Read the model definition and answer for the solid it produces. Units are mm, in the model's axes. Face numbers are marked on the shaded views. A direction names the side the tool comes from. Coordinates: 2 decimals unless noted, no trailing zeros. Loops run counter-clockwise (first coordinate to the right, second up) from the corner with the lowest first, then second, coordinate; pieces in that order, holes last. Notation, with made-up numbers: (49.25, 30) -> (93.25, 30) arc R26 cw to (93.25, 45) -> close; hole circle Ø3 at (58.5, 59.5). An arc over 180 degrees is marked (long way). Answer as a JSON object with one key per item and string values. Group by question number.
Q1. For the marked faces 1, 2 and 3, determine the directions among +Z, -Z, +X, -X, +Y, -Y from which every point of the face is accessible in a straight line to the end or side of a thin tool.
Q2. The part is cut by section A-A on y = 1. Write down the section's boundary in (x, z).
Q3. The part is cut by section D-D on z = 25.5. Write down the section's boundary in (x, y), and give its area (3 significant figures).
Q4. The part is cut by section C-C on x = 0. Write down the section's boundary in (y, z), and give its area (3 significant figures).
Q5. Straight lines are drawn through the part: line 1 along X through (y, z) = (2.45, 2.5); line 2 along Z through (x, y) = (1.75, 1.25); line 3 along X through (y, z) = (0.75, 23). For each, find the intervals that lie inside material, in ascending order. Write a range as [from, to].
Q6. The part is cut by section B-B on z = 9. Write down the section's boundary in (x, y), and give its area (3 significant figures).
Q7. Each of these flat-tipped pins is pushed along its axis until it touches: P1, Ø1.5, axis at x = 8, y = 4, coming from the +Z side; P2, Ø1.2, axis at x = 0, z = 2.5, coming from the +Y side; P3, Ø2.5, axis at y = 4.5, z = 19.5, coming from the -X side; P4, Ø1.5, axis at y = 4, z = 17, coming from the +X side. Where does it stop, or does it pass through?
Q8. Determine the mould class of the marked faces 4, 5 and 6 for opening direction X: released by +X, released by -X, zero draft, split by the parting line, or undercut.
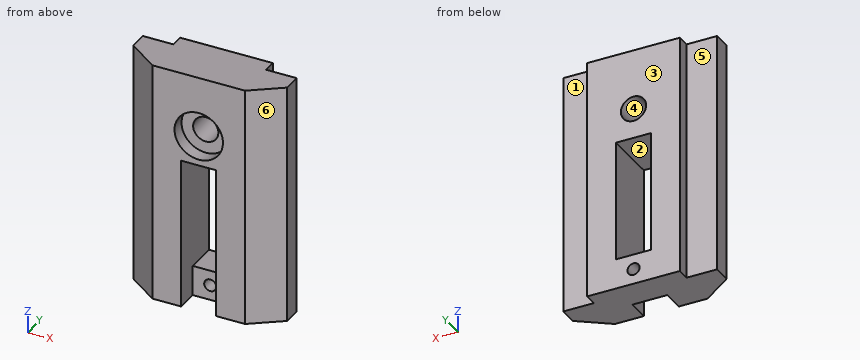
from build123d import *

# Parameters (mm, degrees)
BOSS_EXTRUDE1_DEPTH = 40
SKETCH2_R           = 2.0828
SKETCH2_R_2         = 1
CUT_EXTRUDE1_DEPTH  = 43.867462538
SKETCH3_W           = 5.776667402
SKETCH3_H           = 20
CUT_EXTRUDE2_DEPTH  = 43.867462538
SKETCH4_W           = 5.776667402
SKETCH4_H           = 5
CUT_EXTRUDE3_DEPTH  = 3.62
SKETCH5_R           = 4.0005
CUT_EXTRUDE4_DEPTH  = 2.2098


with BuildPart() as part:
    # Sketch1 → Boss-Extrude1 (new body)
    with BuildSketch(Plane.XY):
        Polygon((-7.65, 5.116666667), (7.65, 5.116666667), (7.65, 3), (12.7, 3), (12.7, 0), (7.65, -3.62), (-7.65, -3.62), (-12.7, 0), (-12.7, 3), (-7.65, 3), align=None)
    extrude(amount=BOSS_EXTRUDE1_DEPTH)

    # Sketch2 → Cut-Extrude1 (cut, through all)
    with BuildSketch(Plane.XZ.offset(3.62)):
        with Locations(Location((0, 30, 0), (0, 0, 270))):
            Circle(SKETCH2_R)
        with Locations(Location((0, 2.5, 0), (0, 0, 270))):
            Circle(SKETCH2_R_2)
    extrude(amount=-CUT_EXTRUDE1_DEPTH, mode=Mode.SUBTRACT)

    # Sketch3 → Cut-Extrude2 (cut, through all)
    with BuildSketch(Plane.XZ.offset(3.62)):
        with Locations((0, 15)):
            Rectangle(SKETCH3_W, SKETCH3_H)
    extrude(amount=-CUT_EXTRUDE2_DEPTH, mode=Mode.SUBTRACT)

    # Sketch4 → Cut-Extrude3 (cut)
    with BuildSketch(Plane.XZ.offset(3.62)):
        with Locations((0, 2.5)):
            Rectangle(SKETCH4_W, SKETCH4_H)
    extrude(amount=-CUT_EXTRUDE3_DEPTH, mode=Mode.SUBTRACT)

    # Sketch5 → Cut-Extrude4 (cut)
    with BuildSketch(Plane.XZ.offset(3.62)):
        with Locations(Location((0, 30, 0), (0, 0, 270))):
            Circle(SKETCH5_R)
    extrude(amount=-CUT_EXTRUDE4_DEPTH, mode=Mode.SUBTRACT)


solid = part.part
Final values:
{
 "1": {"face 1": "+Z, -Z, +X, +Y", "face 2": "+Y, -Y", "face 3": "+Z, -Z, +X, -X, +Y"},
 "2": {"outline": "(-12.7, 0) -> (12.7, 0) -> (12.7, 40) -> (-12.7, 40) -> close; hole (-2.89, 5) -> (2.89, 5) -> (2.89, 25) -> (-2.89, 25) -> close; hole circle Ø4.17 at (0, 30); hole circle Ø2 at (0, 2.5)"},
 "3": {"outline": "(-12.7, 0) -> (-7.65, -3.62) -> (7.65, -3.62) -> (12.7, 0) -> (12.7, 3) -> (7.65, 3) -> (7.65, 5.12) -> (-7.65, 5.12) -> (-7.65, 3) -> (-12.7, 3) -> close", "area": "182 mm2"},
 "4": {"outline": "(-3.62, 25) -> (5.12, 25) -> (5.12, 27.92) -> (-1.41, 27.92) -> (-1.41, 26) -> (-3.62, 26) -> close; (-3.62, 34) -> (-1.41, 34) -> (-1.41, 32.08) -> (5.12, 32.08) -> (5.12, 40) -> (-3.62, 40) -> close; (0, 0) -> (5.12, 0) -> (5.12, 1.5) -> (0, 1.5) -> close; (0, 3.5) -> (5.12, 3.5) -> (5.12, 5) -> (0, 5) -> close", "area": "102 mm2"},
 "5": {"line 1": "x = [-12.7, -1], [1, 12.7]", "line 2": "z = [0, 5], [25, 28.87], [31.13, 40]", "line 3": "x = [-12.7, -2.89], [2.89, 12.7]"},
 "6": {"outline": "(-12.7, 0) -> (-7.65, -3.62) -> (-2.89, -3.62) -> (-2.89, 5.12) -> (-7.65, 5.12) -> (-7.65, 3) -> (-12.7, 3) -> close; (2.89, -3.62) -> (7.65, -3.62) -> (12.7, 0) -> (12.7, 3) -> (7.65, 3) -> (7.65, 5.12) -> (2.89, 5.12) -> close", "area": "132 mm2"},
 "7": {"P1": "stops at z = 40", "P2": "passes through", "P3": "stops at x = -7.65", "P4": "stops at x = 7.65"},
 "8": {"face 4": "undercut", "face 5": "zero draft", "face 6": "released by +X"}
}
